Model file for the job. Use its own axes, mm. A direction names the side the tool comes from. Round coordinates to 2 decimals unless told otherwise and drop trailing zeros. Order: outer loops, then holes, each group sorted by start corner. A loop starts at its lowest first (then second) coordinate and runs counter-clockwise, first axis right, second up. Notation, with made-up numbers: (1, 11.5) - (10, 11.5) arc R10 cw to (10, 19.5) - close; hole circle Ø1 at (-33.5, -23.75). An arc over 180 degrees is marked (long way). Answer as CSV lines item,"result". Start each with the question number.
1. 3-axis set-ups, long thin cutter, end or side, ignore diameter. For faces 1 (the face through (-1, 0, -1)), 2 (the face through (-16.36, 2.18, 13.97)), 3 (the face through (44.126, 5.411, 0.552)): which of +Z, -Z, +X, -X, +Y, -Y reach the whole face in a straight line?
2. Band-saw the part on C-C on y = 2.5. List the corners of the cut face in (x, z).
3. Pin check, flat tip, straight feed: pin 1 Ø12 at (x, z) = (1, -8) entering from -Y. Stop position of the tip, or through.
4. Wall check: line 1 along Z through (x, y) = (-30, 5.75); line 2 along Z through (x, y) = (3.5, 3.75); line 3 along Y through (x, z) = (37, 2). Give the ranges that are in metal, low to high. Write a range as [from, to].
5. Pull direction Z, two halves, no side cores. Call faces 4 (the face through (-1, 3, -38.1)), 5 (the face through (-1, 3, 38.1)), 6 (the face through (-16.364, 2.225, -13.923)): released by +Z, released by -Z, zero draft, split by the parting line, or undercut.
```python
from build123d import *

# Parameters (mm, degrees)
SKETCH1_W            = 101.6
SKETCH1_H            = 76.2
BASE_PLATE_DEPTH     = 6.35
PIPE_START           = -50.8
PIPE_PROFILE_DEPTH   = 69.85
PIPE_PROFILE_2_ANGLE = 180


with BuildPart() as part:
    # Sketch1 → Base Plate (new body)
    with BuildSketch(Plane(origin=(0, 0, 0), x_dir=(1, 0, 0), z_dir=(0, 1, 0))):
        Rectangle(SKETCH1_W, SKETCH1_H)
    extrude(amount=BASE_PLATE_DEPTH)

    # Pipe Profile: read off the stored shape, not the designer's step
    # Pipe Profile outline → Pipe Profile (cut)
    with BuildSketch(Plane.YZ.offset(PIPE_START)):
        with BuildLine():
            Line((6.35, 25.0825), (4.445, 25.0825))
            ThreePointArc((4.445, 25.0825), (2.19993597, 24.15256403), (1.27, 21.9075))
            Line((1.27, 21.9075), (1.27, 16.1925))
            ThreePointArc((1.27, 16.1925), (2.19993597, 13.94743597), (4.445, 13.0175))
            Line((4.445, 13.0175), (6.35, 13.0175))
            Line((6.35, 13.0175), (6.35, 25.0825))
        make_face()
        with BuildLine():
            Line((6.35, -25.0825), (6.35, -13.0175))
            Line((6.35, -13.0175), (4.445, -13.0175))
            ThreePointArc((4.445, -13.0175), (2.19993597, -13.94743597), (1.27, -16.1925))
            Line((1.27, -16.1925), (1.27, -21.9075))
            ThreePointArc((1.27, -21.9075), (2.19993597, -24.15256403), (4.445, -25.0825))
            Line((4.445, -25.0825), (6.35, -25.0825))
        make_face()
    extrude(amount=PIPE_PROFILE_DEPTH, mode=Mode.SUBTRACT)

    # Pipe Profile 2 outline → Pipe Profile 2 (revolve, cut)
    with BuildSketch(Plane.ZY.offset(-19.05)):
        with BuildLine():
            ThreePointArc((13.0175, 4.445), (13.94743597, 2.19993597), (16.1925, 1.27))
            Line((16.1925, 1.27), (21.9075, 1.27))
            ThreePointArc((21.9075, 1.27), (24.15256403, 2.19993597), (25.0825, 4.445))
            Line((25.0825, 4.445), (25.0825, 6.35))
            Line((25.0825, 6.35), (13.0175, 6.35))
            Line((13.0175, 6.35), (13.0175, 4.445))
        make_face()
    revolve(axis=Axis((19.05, 0, 0), (0, 1, 0)), revolution_arc=PIPE_PROFILE_2_ANGLE, mode=Mode.SUBTRACT)


solid = part.part
```
Reply:
1,face 1,"+Z, -Z, +X, -X, -Y"
1,face 2,"-X, +Y"
1,face 3,"+Y"
2,outline,"(-50.8, -38.1) - (50.8, -38.1) - (50.8, 38.1) - (-50.8, 38.1) - (-50.8, 24.42) - (19.05, 24.42) arc R24.42 cw to (19.05, -24.42) - (-50.8, -24.42) - close; (-50.8, -13.68) - (19.05, -13.68) arc R13.68 ccw to (19.05, 13.68) - (-50.8, 13.68) - close"
3,pin 1,"stops at y = 0"
4,line 1,"z = [-38.1, -25.08], [-13.02, 13.02], [25.08, 38.1]"
4,line 2,"z = [-38.1, -25.01], [-13.09, 13.09], [25.01, 38.1]"
4,line 3,"y = [0, 1.27]"
5,face 4,"released by -Z"
5,face 5,"released by +Z"
5,face 6,"undercut"
